Source: CAD feature listing. Evaluate the final solid. Frame: model axes, mm. Face numbers are marked on the shaded views. Give positions to 0.01 mm unless a question says otherwise; leave off trailing zeros. Order: outer loops, then holes, each group sorted by start corner. A loop starts at its lowest first (then second) coordinate and runs counter-clockwise, first axis right, second up.
```python
from build123d import *

# Parameters (mm, degrees)
F0_R        = 14
F0_R_2      = 5
F1_DEPTH    = 3
F0_R_3      = 15
F1_FACE_R   = 14
F1_FACE_R_2 = 5
F2_DEPTH    = 0.5


with BuildPart() as f1:
    # F0 (on Top) → F1 (new body)
    with BuildSketch(Plane.XY):
        Circle(F0_R)
        with Locations((6.601435598, 0)):
            Circle(F0_R_2, mode=Mode.SUBTRACT)
    extrude(amount=F1_DEPTH)

    # F0 (on Top) + F1_face (on face) → F2 (join)
    with BuildSketch(Plane.XY):
        Circle(F0_R_3)
        Circle(F0_R, mode=Mode.SUBTRACT)
        Circle(F0_R)
        with Locations((6.601435598, 0)):
            Circle(F0_R_2, mode=Mode.SUBTRACT)
        with Locations((6.601435598, 0)):
            Circle(F0_R_2)
    with BuildSketch(Plane(origin=(-0.9651221634, 0, 3), x_dir=(1, 0, 0), z_dir=(0, 0, 1))):
        with Locations((0.9651221634, 0)):
            Circle(F1_FACE_R)
        with Locations((7.5665577614, 0)):
            Circle(F1_FACE_R_2, mode=Mode.SUBTRACT)
    extrude(amount=-F2_DEPTH)


solid = f1.part
```
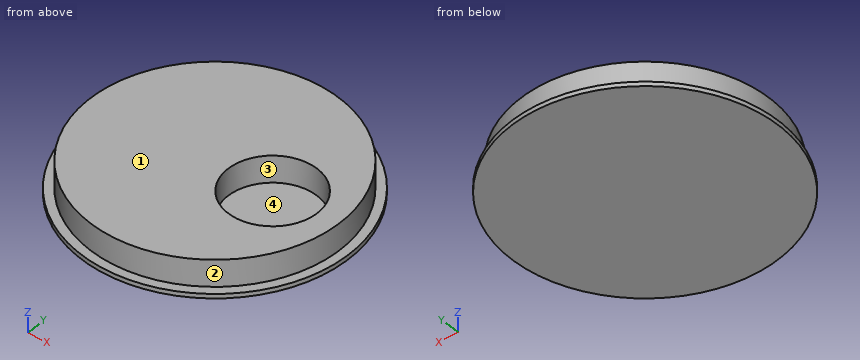
1) Section query A-A, the plane x = 0. Return the cut outline in (y, z).
Report:
outline: (-15, -0.5) - (15, -0.5) - (15, 0) - (14, 0) - (14, 3) - (-14, 3) - (-14, 0) - (-15, 0) - close
2) Draft query along Y for the marked faces 1, 2, 3 and 4. Return one class per face: +Y half, -Y half, draft (parallel to the pull), parting line (faces both ways), or undercut.
Report:
face 1: draft
face 2: parting line
face 3: undercut
face 4: undercut
3) Section query B-B, the plane y = 0. Return the cut outline in (x, z), and give its area (3 significant figures).
Report:
outline: (-15, -0.5) - (15, -0.5) - (15, 0) - (14, 0) - (14, 3) - (11.6, 3) - (11.6, 0) - (1.6, 0) - (1.6, 3) - (-14, 3) - (-14, 0) - (-15, 0) - close
area: 69.0 mm2
4) Pin query (flat end, axial travel): pin 1 (5 mm diameter, centred on x = 7, y = -1, fed in from +Z); pin 2 (1.5 mm diameter, centred on y = 0.5, z = 2.5, fed in from +X). Return the tip coordinate at first contact, or that it passes through.
Report:
pin 1: stops at z = 0
pin 2: stops at x = 14
5) Section query D-D, the plane x = -7.5. Return the cut outline in (y, z).
Report:
outline: (-12.99, -0.5) - (12.99, -0.5) - (12.99, 0) - (11.82, 0) - (11.82, 3) - (-11.82, 3) - (-11.82, 0) - (-12.99, 0) - close
6) Material intervals for L1, parallel to Y at x = 4, z = 0.3; L2, parallel to Z at x = 9.25, y = 0.25; L3, parallel to Y at x = 3.5, z = 0.3, sorted ascending.
Report:
L1: y = -13.42 to -4.27, 4.27 to 13.42
L2: z = -0.5 to 0
L3: y = -13.56 to -3.92, 3.92 to 13.56
7) Section query C-C, the plane z = 2.2. Return the cut outline in (x, y), and give its area (3 significant figures).
Report:
outline: circle Ø28 at (0, 0); hole circle Ø10 at (6.6, 0)
area: 537 mm2
